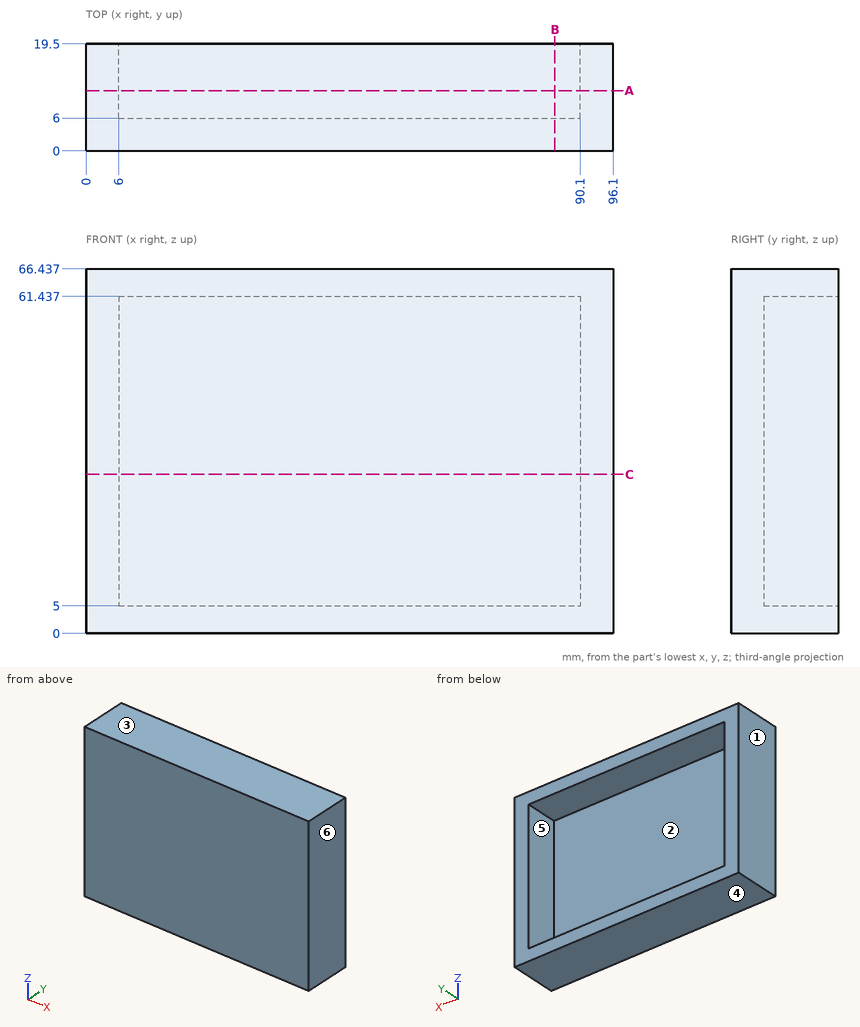
Input: dimensioned drawing with shaded views. Units: mm. Origin: part minimum x, y, z. A direction names the side the tool comes from. Coordinates: 2 decimals unless noted, no trailing zeros. Order: outer loops, then holes, each group sorted by start corner. A loop starts at its lowest first (then second) coordinate and runs counter-clockwise, first axis right, second up.
Item 1: Draft query along Z for the marked faces 3, 4, 5 and 6. Return one class per face: released by +Z, released by -Z, zero draft, split by the parting line, or undercut.
Answer:
face 3: released by +Z
face 4: released by -Z
face 5: undercut
face 6: zero draft
Item 2: Contact query for a flat-ended pin moving along its axis: P1, Ø2, axis at x = 40, z = 46.5, coming from the +Y side. Output: stop coordinate, or through.
Answer:
P1: stops at y = 6
Item 3: Access query for the marked faces 1 and 2. Directions: +Z, -Z, +X, -X, +Y, -Y. A direction counts if a zero-diameter tool reaches every point of the face in a straight line with its end or side. Return the directions, or none.
Answer:
face 1: +Z, -Z, -X, +Y, -Y
face 2: +Y
Item 4: Section query A-A (y = 11). Output: boundary loops of the cut face in (x, z).
Answer:
outline: (0, 0) - (96.1, 0) - (96.1, 66.44) - (0, 66.44) - close; hole (6, 5) - (90.1, 5) - (90.1, 61.44) - (6, 61.44) - close
Item 5: Section query C-C (z = 29). Output: boundary loops of the cut face in (x, y).
Answer:
outline: (0, 0) - (96.1, 0) - (96.1, 19.5) - (90.1, 19.5) - (90.1, 6) - (6, 6) - (6, 19.5) - (0, 19.5) - close
Item 6: Material intervals for line 1 along X through (y, z) = (12.5, 30.5); line 2 along Z through (x, y) = (46.5, 7.25); line 3 along Y through (x, z) = (30, 17.5), sorted ascending.
Answer:
line 1: x = 0 to 6, 90.1 to 96.1
line 2: z = 0 to 5, 61.44 to 66.44
line 3: y = 0 to 6
Item 7: Section query B-B (x = 85.5). Output: boundary loops of the cut face in (y, z).
Answer:
outline: (0, 0) - (19.5, 0) - (19.5, 5) - (6, 5) - (6, 61.44) - (19.5, 61.44) - (19.5, 66.44) - (0, 66.44) - close
